```python
from build123d import *

# Parameters (mm, degrees)
ESTRUSIONE_ESTRUSIONE1_DEPTH = 5
TAGLIO_ESTRUSIONE5_DEPTH     = 6
SCHIZZO2_W                   = 5
SCHIZZO2_H                   = 37.5
TAGLIO_ESTRUSIONE1_DEPTH     = 6
SCHIZZO3_R                   = 1.5
TAGLIO_ESTRUSIONE2_DEPTH     = 6
SCHIZZO8_W                   = 7
SCHIZZO8_H                   = 7
TAGLIO_ESTRUSIONE6_DEPTH     = 6
SCHIZZO10_R                  = 0.25
TAGLIO_ESTRUSIONE11_DEPTH    = 6


with BuildPart() as part:
    # Schizzo1 → Estrusione-Estrusione1 (new body)
    with BuildSketch(Plane(origin=(0, 0, 0), x_dir=(0, 0, -1), z_dir=(1, 0, 0))):
        Polygon((165, 60), (-106.353966324, 60), (-165, 10), (-165, -60), (165, -60), align=None)
    extrude(amount=ESTRUSIONE_ESTRUSIONE1_DEPTH)

    # Schizzo7 → Taglio-Estrusione5 (cut, through all)
    with BuildSketch(Plane(origin=(0, 0, 0), x_dir=(0, 0, -1), z_dir=(1, 0, 0))):
        Polygon((165, 40), (165, 60), (120.869304328, 60), align=None)
    extrude(amount=TAGLIO_ESTRUSIONE5_DEPTH, mode=Mode.SUBTRACT)

    # Schizzo2 → Taglio-Estrusione1 (cut, through all)
    with BuildSketch(Plane(origin=(5, 0, 0), x_dir=(0, 0, -1), z_dir=(1, 0, 0))):
        with Locations((100, -41.25)):
            Rectangle(SCHIZZO2_W, SCHIZZO2_H)
        with Locations((0, -41.25)):
            Rectangle(SCHIZZO2_W, SCHIZZO2_H)
        with Locations((-100, -41.25)):
            Rectangle(SCHIZZO2_W, SCHIZZO2_H)
    extrude(amount=-TAGLIO_ESTRUSIONE1_DEPTH, mode=Mode.SUBTRACT)

    # Schizzo3 → Taglio-Estrusione2 (cut, through all)
    with BuildSketch(Plane(origin=(0, 0, 0), x_dir=(0, 0, -1), z_dir=(1, 0, 0))):
        with Locations((-65.12, 55)):
            Circle(SCHIZZO3_R)
        with Locations((-18.62, 55)):
            Circle(SCHIZZO3_R)
        with Locations((-95.12, 55)):
            Circle(SCHIZZO3_R)
        with Locations((21.38, 55)):
            Circle(SCHIZZO3_R)
        with Locations((61.38, 55)):
            Circle(SCHIZZO3_R)
        with Locations((101.38, 55)):
            Circle(SCHIZZO3_R)
        with Locations((-118.329493742, 43.219453434)):
            Circle(SCHIZZO3_R)
        with Locations((-146.536630365, 19.170822303)):
            Circle(SCHIZZO3_R)
        with Locations((-160, -10)):
            Circle(SCHIZZO3_R)
        with Locations((-160, -40)):
            Circle(SCHIZZO3_R)
        with Locations((160, -40)):
            Circle(SCHIZZO3_R)
        with Locations((160, 20)):
            Circle(SCHIZZO3_R)
        with Locations((140.870719583, 45.44586097)):
            Circle(SCHIZZO3_R)
        with BuildLine():
            Line((-60.87, 26.5), (-60.87, 60))
            ThreePointArc((-60.87, 60), (-41.87, 79), (-22.87, 60))
            Line((-22.87, 60), (-22.87, 26.5))
            ThreePointArc((-22.87, 26.5), (-41.87, 7.5), (-60.87, 26.5))
        make_face()
    extrude(amount=TAGLIO_ESTRUSIONE2_DEPTH, mode=Mode.SUBTRACT)

    # Schizzo8 → Taglio-Estrusione6 (cut, through all)
    with BuildSketch(Plane(origin=(5, 0, 0), x_dir=(0, 0, -1), z_dir=(1, 0, 0))):
        with Locations((0, -56.5)):
            Rectangle(SCHIZZO8_W, SCHIZZO8_H)
        with Locations((100, -56.5)):
            Rectangle(SCHIZZO8_W, SCHIZZO8_H)
        with Locations((-100, -56.5)):
            Rectangle(SCHIZZO8_W, SCHIZZO8_H)
    extrude(amount=-TAGLIO_ESTRUSIONE6_DEPTH, mode=Mode.SUBTRACT)

    # Schizzo10 → Taglio-Estrusione11 (cut, through all)
    with BuildSketch(Plane(origin=(0, 0, 0), x_dir=(0, 0, -1), z_dir=(1, 0, 0))):
        with Locations((-102.5, -22.5)):
            Circle(SCHIZZO10_R)
        with Locations((-97.5, -22.5)):
            Circle(SCHIZZO10_R)
        with Locations((-103.5, -53)):
            Circle(SCHIZZO10_R)
        with Locations((-96.5, -53)):
            Circle(SCHIZZO10_R)
        with Locations((-2.5, -22.5)):
            Circle(SCHIZZO10_R)
        Circle(SCHIZZO10_R)
        with Locations((2.5, -22.5)):
            Circle(SCHIZZO10_R)
        with Locations((-3.5, -53)):
            Circle(SCHIZZO10_R)
        with Locations((3.5, -53)):
            Circle(SCHIZZO10_R)
        with Locations((97.5, -22.5)):
            Circle(SCHIZZO10_R)
        with Locations((102.5, -22.5)):
            Circle(SCHIZZO10_R)
        with Locations((96.5, -53)):
            Circle(SCHIZZO10_R)
        with Locations((103.5, -53)):
            Circle(SCHIZZO10_R)
    extrude(amount=TAGLIO_ESTRUSIONE11_DEPTH, mode=Mode.SUBTRACT)


solid = part.part
```
Here's how the part is built. I have some questions about the finished solid (model axes, mm). Round coordinates to 2 decimals unless told otherwise and drop trailing zeros. Order: outer loops, then holes, each group sorted by start corner. A loop starts at its lowest first (then second) coordinate and runs counter-clockwise, first axis right, second up. Notation, with made-up numbers: M 34.25,-6.75 L 43.25,-6.75 A11 cw 43.25,-1.75 Z; hole C 64,-23.75 d2. An arc over 180 degrees is marked long. Use CSV: the item, a comma, the result in double quotes.
1) If we mould it in two halves opening along Z, with no side actions, what happens to faces 1 (the flat face through (2.465, 35.35, 135.266)), 2 (the flat face through (5, 1, 2)), 3 (the cylindrical face through (2.465, 7.505, 41.452))? For each: pulls with the +Z half, pulls with the -Z half, needs draft (parallel to the pull), parting line crosses it, or undercut.
Taken from the geometry:
face 1,"pulls with the +Z half"
face 2,"needs draft"
face 3,"undercut"
2) I'm going to push flat-ended pins straight in: P1, Ø1, axis at x = 4, z = -124, coming from the +Y side; P2, Ø1.8, axis at y = 55, z = 65.12, coming from the -X side; P3, Ø4, axis at y = -10, z = 160, coming from the +X side; P4, Ø1, axis at x = 3.5, y = 12.5, coming from the +Z side. Where does each tip first touch, or does it pass through?
Taken from the geometry:
P1,"y = 58.81"
P2,"through"
P3,"x = 5"
P4,"z = 162.65"
3) I want a section at A-A (y = -29.5). List the corners of the cut face in (x, z) for me.
Taken from the geometry:
outline,"M 0,-165 L 5,-165 L 5,-102.5 L 0,-102.5 Z; M 0,-97.5 L 5,-97.5 L 5,-2.5 L 0,-2.5 Z; M 0,2.5 L 5,2.5 L 5,97.5 L 0,97.5 Z; M 0,102.5 L 5,102.5 L 5,165 L 0,165 Z"
4) I want a section at B-B (y = 32). List the corners of the cut face in (x, z) for me.
Taken from the geometry:
outline,"M 0,-165 L 5,-165 L 5,22.87 L 0,22.87 Z; M 0,60.87 L 5,60.87 L 5,139.2 L 0,139.2 Z"
5) I need wall thicknesses on line 1 along Z through (x, y) = (0.25, -54); line 2 along Z through (x, y) = (3.3, -31.5); line 3 along Z through (x, y) = (2.65, -41). Which ranges of each line are inside material? Lowest first, please. Write a range as [from, to].
Taken from the geometry:
line 1,"[-165, -103.5], [-96.5, -3.5], [3.5, 96.5], [103.5, 165]"
line 2,"[-165, -102.5], [-97.5, -2.5], [2.5, 97.5], [102.5, 165]"
line 3,"[-165, -161.12], [-158.88, -102.5], [-97.5, -2.5], [2.5, 97.5], [102.5, 158.88], [161.12, 165]"
6) I want a section at D-D (z = 110). List the corners of the cut face in (x, y) for me.
Taken from the geometry:
outline,"M 0,-60 L 5,-60 L 5,56.89 L 0,56.89 Z"
7) I want a section at C-C (x = 3.4). Count the separate pieces of the cut face and the enclosed holes in it, then the cut area to 3 significant figures.
Taken from the geometry:
separate pieces,"1"
enclosed holes,"14"
area,"35,200 mm^2"
